from build123d import *

# Parameters (mm, degrees)
F0_R     = 2.1
F1_DEPTH = 200
F2_R     = 2.1
F3_DEPTH = 7
F4_R     = 1.6
F5_DEPTH = 7


with BuildPart() as f1:
    # F0 (on Top) → F1 (new body)
    with BuildSketch(Plane.XY):
        with BuildLine():
            ThreePointArc((-3.308023, 10.226634), (-3.381246, 10.403411), (-3.558023, 10.476634))
            Line((-3.558023, 10.476634), (-10.308023, 10.476634))
            ThreePointArc((-10.308023, 10.476634), (-10.499365, 10.438574), (-10.661577, 10.330188))
            ThreePointArc((-10.661577, 10.330188), (-10.769963, 10.167976), (-10.808023, 9.976634))
            Line((-10.808023, 9.976634), (-10.808023, 3.226634))
            ThreePointArc((-10.808023, 3.226634), (-10.7348, 3.049858), (-10.558023, 2.976634))
            Line((-10.558023, 2.976634), (-9.555049, 2.976634))
            ThreePointArc((-9.555049, 2.976634), (-9.378272, 3.049858), (-9.305049, 3.226634))
            Line((-9.305049, 3.226634), (-9.305049, 6.654412))
            ThreePointArc((-9.305049, 6.654412), (-9.024273, 7.159685), (-8.45447, 7.062421))
            Line((-8.45447, 7.062421), (-4.381246, 2.989198))
            ThreePointArc((-4.381246, 2.989198), (-4.327053, 2.908092), (-4.308023, 2.812421))
            Line((-4.308023, 2.812421), (-4.308023, -1.859152))
            ThreePointArc((-4.308023, -1.859152), (-4.327053, -1.954823), (-4.381246, -2.035929))
            Line((-4.381246, -2.035929), (-8.45447, -6.109152))
            ThreePointArc((-8.45447, -6.109152), (-8.999365, -6.217538), (-9.308023, -5.755599))
            Line((-9.308023, -5.755599), (-9.308023, -2.273366))
            ThreePointArc((-9.308023, -2.273366), (-9.381246, -2.096589), (-9.558023, -2.023366))
            Line((-9.558023, -2.023366), (-10.558023, -2.023366))
            ThreePointArc((-10.558023, -2.023366), (-10.7348, -2.096589), (-10.808023, -2.273366))
            Line((-10.808023, -2.273366), (-10.808023, -9.023366))
            ThreePointArc((-10.808023, -9.023366), (-10.769963, -9.214707), (-10.661577, -9.376919))
            ThreePointArc((-10.661577, -9.376919), (-10.508248, -9.481525), (-10.327327, -9.522993))
            Line((-10.327327, -9.522993), (-3.544376, -9.522993))
            ThreePointArc((-3.544376, -9.522993), (-3.376486, -9.44525), (-3.308023, -9.273366))
            Line((-3.308023, -9.273366), (-3.308023, -8.273366))
            ThreePointArc((-3.308023, -8.273366), (-3.381246, -8.096589), (-3.558023, -8.023366))
            Line((-3.558023, -8.023366), (-7.040256, -8.023366))
            ThreePointArc((-7.040256, -8.023366), (-7.502196, -7.714707), (-7.39381, -7.169812))
            Line((-7.39381, -7.169812), (-3.320586, -3.096589))
            ThreePointArc((-3.320586, -3.096589), (-3.23948, -3.042396), (-3.14381, -3.023366))
            Line((-3.14381, -3.023366), (1.527763, -3.023366))
            ThreePointArc((1.527763, -3.023366), (1.623434, -3.042396), (1.70454, -3.096589))
            Line((1.70454, -3.096589), (5.777763, -7.169812))
            ThreePointArc((5.777763, -7.169812), (5.88615, -7.714707), (5.42421, -8.023366))
            Line((5.42421, -8.023366), (1.95454, -8.023366))
            ThreePointArc((1.95454, -8.023366), (1.777763, -8.096589), (1.70454, -8.273366))
            Line((1.70454, -8.273366), (1.70454, -9.273366))
            ThreePointArc((1.70454, -9.273366), (1.773002, -9.44525), (1.940893, -9.522993))
            Line((1.940893, -9.522993), (8.711281, -9.522993))
            ThreePointArc((8.711281, -9.522993), (8.892202, -9.481525), (9.04553, -9.376919))
            ThreePointArc((9.04553, -9.376919), (9.141878, -9.241515), (9.188525, -9.082012))
            Line((9.188525, -9.082012), (9.188525, -2.231968))
            ThreePointArc((9.188525, -2.231968), (9.103455, -2.082513), (8.941977, -2.023366))
            Line((8.941977, -2.023366), (7.941977, -2.023366))
            ThreePointArc((7.941977, -2.023366), (7.7652, -2.096589), (7.691977, -2.273366))
            Line((7.691977, -2.273366), (7.691977, -5.755599))
            ThreePointArc((7.691977, -5.755599), (7.383319, -6.217538), (6.838423, -6.109152))
            Line((6.838423, -6.109152), (2.7652, -2.035929))
            ThreePointArc((2.7652, -2.035929), (2.711007, -1.954823), (2.691977, -1.859152))
            Line((2.691977, -1.859152), (2.691977, 2.812421))
            ThreePointArc((2.691977, 2.812421), (2.711007, 2.908092), (2.7652, 2.989198))
            Line((2.7652, 2.989198), (6.838423, 7.062421))
            ThreePointArc((6.838423, 7.062421), (7.383319, 7.170807), (7.691977, 6.708867))
            Line((7.691977, 6.708867), (7.691977, 3.226634))
            ThreePointArc((7.691977, 3.226634), (7.7652, 3.049858), (7.941977, 2.976634))
            Line((7.941977, 2.976634), (8.941977, 2.976634))
            ThreePointArc((8.941977, 2.976634), (9.103455, 3.035782), (9.188525, 3.185237))
            Line((9.188525, 3.185237), (9.188525, 10.035281))
            ThreePointArc((9.188525, 10.035281), (9.141878, 10.194784), (9.04553, 10.330188))
            ThreePointArc((9.04553, 10.330188), (8.883319, 10.438574), (8.691977, 10.476634))
            Line((8.691977, 10.476634), (1.941977, 10.476634))
            ThreePointArc((1.941977, 10.476634), (1.7652, 10.403411), (1.691977, 10.226634))
            Line((1.691977, 10.226634), (1.691977, 9.226634))
            ThreePointArc((1.691977, 9.226634), (1.695138, 9.187006), (1.70454, 9.14838))
            ThreePointArc((1.70454, 9.14838), (1.795456, 9.024071), (1.941977, 8.976634))
            Line((1.941977, 8.976634), (5.42421, 8.976634))
            ThreePointArc((5.42421, 8.976634), (5.88615, 8.667976), (5.777763, 8.123081))
            Line((5.777763, 8.123081), (1.70454, 4.049858))
            ThreePointArc((1.70454, 4.049858), (1.623434, 3.995664), (1.527763, 3.976634))
            Line((1.527763, 3.976634), (-3.14381, 3.976634))
            ThreePointArc((-3.14381, 3.976634), (-3.23948, 3.995664), (-3.320586, 4.049858))
            Line((-3.320586, 4.049858), (-7.39381, 8.123081))
            ThreePointArc((-7.39381, 8.123081), (-7.502196, 8.667976), (-7.040256, 8.976634))
            Line((-7.040256, 8.976634), (-3.558023, 8.976634))
            ThreePointArc((-3.558023, 8.976634), (-3.381246, 9.049858), (-3.308023, 9.226634))
            Line((-3.308023, 9.226634), (-3.308023, 9.726634))
            Line((-3.308023, 9.726634), (-3.308023, 10.226634))
        make_face()
        with Locations((-0.808023, 0.476634)):
            Circle(F0_R, mode=Mode.SUBTRACT)
    extrude(amount=F1_DEPTH)

    # F2 (on face) → F3 (cut)
    with BuildSketch(Plane.YZ.offset(2.691977)):
        with Locations((0.476634, 79.99858)):
            Circle(F2_R)
    extrude(amount=-F3_DEPTH, mode=Mode.SUBTRACT)

    # F4 (on face) → F5 (cut)
    with BuildSketch(Plane(origin=(0, 3.976634, 0), x_dir=(-1, 0, 0), z_dir=(0, 1, 0))):
        with Locations((0.808023, 190)):
            Circle(F4_R)
    extrude(amount=-F5_DEPTH, mode=Mode.SUBTRACT)


solid = f1.part
Source: CAD feature listing. Evaluate the final solid. Frame: model axes, mm. A direction names the side the tool comes from. Give positions to 0.01 mm unless a question says otherwise; leave off trailing zeros. Return JSON: item names as keys, results as strings. Group by question number.
1) Set-up query: faces 1 (the face through (-1, -3.023, 99)), 2 (the face through (4, -8.023, 99)), 3 (the face through (-4.308, 1, 99)), 4 (the face through (-7, -9.523, 99)), 5 (the face through (-7, 10.477, 99)). Return all of +Z, -Z, +X, -X, +Y, -Y with unobstructed straight access to the full face (end or side cutting, diameter ignored); none if empty.
2) Pull-direction query (X, two-part tool) for faces 6 (the face through (-5, 8.977, 99)), 7 (the face through (2.692, 0, 99)), 8 (the face through (-10.808, -6, 99)); classes: pulls with the +X half, pulls with the -X half, needs draft (parallel to the pull), parting line crosses it, or undercut.
3) Pin query (flat end, axial travel): P1, Ø1.4, axis at y = 1, z = 71, coming from the -X side; P2, Ø1.9, axis at x = -0.81, z = 190, coming from the +Y side (1 decimal). Return the tip coordinate at first contact, or that it passes through.
4) Material intervals for line 1 along X through (y, z) = (-7.5, 65); line 2 along X through (y, z) = (9.5, 60.5); line 3 along Y through (x, z) = (7.25, 22.5), sorted ascending. Write a range as [from, to].
Recorded:
{
 "1": {"face 1": "+Z, -Z, -Y", "face 2": "+Z, -Z", "face 3": "+Z, -Z, -X", "face 4": "+Z, -Z, +X, -X, -Y", "face 5": "+Z, -Z, +X, -X, +Y"},
 "2": {"face 6": "undercut", "face 7": "pulls with the +X half", "face 8": "pulls with the -X half"},
 "3": {"P1": "stops at x = -4.31", "P2": "passes through"},
 "4": {"line 1": "x = [-10.81, -7.54], [5.92, 9.19]", "line 2": "x = [-10.81, -3.31], [1.69, 9.19]", "line 3": "y = [-9.52, -6.25], [7.21, 10.48]"}
}
